Read the model definition and answer for the solid it produces. Units are mm, in the model's axes. Coordinates: 2 decimals unless noted, no trailing zeros. Loops run counter-clockwise (first coordinate to the right, second up) from the corner with the lowest first, then second, coordinate; pieces in that order, holes last.
from build123d import *

# Parameters (mm, degrees)
SKETCH1_W           = 735
SKETCH1_H           = 1240
SKETCH1_W_2         = 655
SKETCH1_H_2         = 1150
BOSS_EXTRUDE1_DEPTH = 6
SKETCH2_W           = 697
SKETCH2_H           = 1192
CUT_EXTRUDE1_DEPTH  = 2


with BuildPart() as part:
    # Sketch1 → Boss-Extrude1 (new body)
    with BuildSketch(Plane(origin=(0, 0, 0), x_dir=(1, 0, 0), z_dir=(0, 1, 0))):
        Rectangle(SKETCH1_W, SKETCH1_H)
        with Locations((0, -5)):
            Rectangle(SKETCH1_W_2, SKETCH1_H_2, mode=Mode.SUBTRACT)
    extrude(amount=BOSS_EXTRUDE1_DEPTH)

    # Sketch2 → Cut-Extrude1 (cut)
    with BuildSketch(Plane.XZ):
        with Locations((0, 5)):
            Rectangle(SKETCH2_W, SKETCH2_H)
    extrude(amount=-CUT_EXTRUDE1_DEPTH, mode=Mode.SUBTRACT)


solid = part.part
Item 1: Find the intervals of material crossed by line 1 along X through (y, z) = (4.3, 490.5); line 2 along X through (y, z) = (1.2, -109); line 3 along Z through (x, y) = (136.5, 4.4), in increasing order.
Numbers:
line 1: x = -367.5 to -327.5, 327.5 to 367.5
line 2: x = -367.5 to -348.5, 348.5 to 367.5
line 3: z = -620 to -570, 580 to 620
Item 2: A cutting plane is placed at B-B on z = -334. Determine the outline of the cut face in (x, y), then the cut area to 3 significant figures.
Numbers:
outline: (-367.5, 0) - (-348.5, 0) - (-348.5, 2) - (-327.5, 2) - (-327.5, 6) - (-367.5, 6) - close; (327.5, 2) - (348.5, 2) - (348.5, 0) - (367.5, 0) - (367.5, 6) - (327.5, 6) - close
area: 396 mm2
Item 3: A cutting plane is placed at C-C on y = 4.8. Determine the outline of the cut face in (x, z).
Numbers:
outline: (-367.5, -620) - (367.5, -620) - (367.5, 620) - (-367.5, 620) - close; hole (-327.5, -570) - (327.5, -570) - (327.5, 580) - (-327.5, 580) - close
Item 4: A cutting plane is placed at A-A on x = 239. Determine the outline of the cut face in (y, z).
Numbers:
outline: (0, -620) - (6, -620) - (6, -570) - (2, -570) - (2, -591) - (0, -591) - close; (0, 601) - (2, 601) - (2, 580) - (6, 580) - (6, 620) - (0, 620) - close
Item 5: Determine the mould class of faces 1 (the face through (-328, 6, -3)), 2 (the face through (334, 2, 184)) for opening direction Z: released by +Z, released by -Z, zero draft, split by the parting line, or undercut.
Numbers:
face 1: zero draft
face 2: undercut
